Build history of the part. All positions in model axes, mm. A direction names the side the tool comes from. Give positions to 0.01 mm unless a question says otherwise; leave off trailing zeros. Loops run counter-clockwise (first coordinate to the right, second up) from the corner with the lowest first, then second, coordinate; pieces in that order, holes last. Notation, with made-up numbers: (8, 49) -> (14, 49) arc R7 cw to (14, 57) -> close; hole circle Ø4 at (0.5, 5). An arc over 180 degrees is marked (long way). Answer as a JSON object with one key per item and string values. Group by question number.
Q1. Band-saw the part on A-A, the plane y = 77.5. Write the cut outline in (x, z).
Q2. Two-plate mould, pull along Z, no slides. Class faces 3 (the flat face through (3.7, 75, -82)), 4 (the flat face through (0.1, 74, -85.4)), 5 (the flat face through (0, 77, -73)): pulls with the +Z half, pulls with the -Z half, needs draft (parallel to the pull), parting line crosses it, or undercut.
Q3. Band-saw the part on B-B, the plane x = 0.5. Write the cut outline in (y, z).
Q4. Drop flat-ended pins along their axis: pin 1 (1 mm diameter, centred on x = -6, y = 77.5, fed in from -Z); pin 2 (3.5 mm diameter, centred on x = 0.5, z = -80.5, fed in from -Y). Give the stop position or say it passes through.
Q5. Tool access for faces 1 (the flat face through (0, 75, -85.2)), 2 (the cylindrical face through (7.6, 76.96, -89.14)): list every direction of +Z, -Z, +X, -X, +Y, -Y with a clear straight run to the whole face (end or side of a thin tool).
Q6. Band-saw the part on C-C, the plane x = -6.75. Write the cut outline in (y, z).
Q7. Wall check: probe 1 along Z at (x, y) = (2.25, 76.35); probe 2 along X at (y, z) = (76.7, -83); probe 3 along Y at (x, z) = (2.5, -81.75). Give the ranges that are in metal, low to high. Write a range as from..to.
from build123d import *

# Parameters (mm, degrees)
CAP_START         = 74
CAP_DEPTH         = 6
STEM_START        = 73.8
STEM_SOCKET_DEPTH = 3.2


with BuildPart() as part:
    # Sketch1 → Cap (new body)
    with BuildSketch(Plane(origin=(0, 0, 0), x_dir=(1, 0, 0), z_dir=(0, 1, 0)).offset(CAP_START)):
        with BuildLine():
            Line((-5.5, 90), (5.5, 90))
            ThreePointArc((5.5, 90), (7.621320344, 89.121320344), (8.5, 87))
            Line((8.5, 87), (8.5, 76))
            ThreePointArc((8.5, 76), (7.621320344, 73.878679656), (5.5, 73))
            Line((5.5, 73), (-5.5, 73))
            ThreePointArc((-5.5, 73), (-7.621320344, 73.878679656), (-8.5, 76))
            Line((-8.5, 76), (-8.5, 87))
            ThreePointArc((-8.5, 87), (-7.621320344, 89.121320344), (-5.5, 90))
        make_face()
    extrude(amount=CAP_DEPTH)

    # Sketch2 → Stem socket (cut)
    with BuildSketch(Plane(origin=(0, 0, 0), x_dir=(1, 0, 0), z_dir=(0, 1, 0)).offset(STEM_START)):
        with BuildLine():
            Line((-3.3, 85.2), (3.3, 85.2))
            ThreePointArc((3.3, 85.2), (3.582842712, 85.082842712), (3.7, 84.8))
            Line((3.7, 84.8), (3.7, 78.2))
            ThreePointArc((3.7, 78.2), (3.582842712, 77.917157288), (3.3, 77.8))
            Line((3.3, 77.8), (-3.3, 77.8))
            ThreePointArc((-3.3, 77.8), (-3.582842712, 77.917157288), (-3.7, 78.2))
            Line((-3.7, 78.2), (-3.7, 84.8))
            ThreePointArc((-3.7, 84.8), (-3.582842712, 85.082842712), (-3.3, 85.2))
        make_face()
    extrude(amount=STEM_SOCKET_DEPTH, mode=Mode.SUBTRACT)


solid = part.part
Worked answers:
{
 "1": {"outline": "(-8.5, -87) arc R3 ccw to (-5.5, -90) -> (5.5, -90) arc R3 ccw to (8.5, -87) -> (8.5, -76) arc R3 ccw to (5.5, -73) -> (-5.5, -73) arc R3 ccw to (-8.5, -76) -> close"},
 "2": {"face 3": "undercut", "face 4": "needs draft", "face 5": "pulls with the +Z half"},
 "3": {"outline": "(74, -90) -> (80, -90) -> (80, -73) -> (74, -73) -> (74, -77.8) -> (77, -77.8) -> (77, -85.2) -> (74, -85.2) -> close"},
 "4": {"pin 1": "z = -90", "pin 2": "y = 77"},
 "5": {"face 1": "-Y", "face 2": "-Z, +X, +Y, -Y"},
 "6": {"outline": "(74, -89.73) -> (80, -89.73) -> (80, -73.27) -> (74, -73.27) -> close"},
 "7": {"probe 1": "-90..-85.2, -77.8..-73", "probe 2": "-8.5..-3.7, 3.7..8.5", "probe 3": "77..80"}
}
